Can you work these out from the model? Positions are in its coordinate system, mm. A direction names the side the tool comes from. Give positions to 0.01 mm unless a question says otherwise; leave off trailing zeros. Order: outer loops, then holes, each group sorted by start corner. A loop starts at its lowest first (then second) coordinate and runs counter-clockwise, first axis right, second up. Notation, with made-up numbers: (21.5, 8) -> (73.5, 8) arc R33 ccw to (73.5, 40) -> close; hole circle Ø4 at (-22.75, 46). An arc over 180 degrees is marked (long way). Answer as a JSON object with one key per item and string values.
```python
from build123d import *

# Parameters (mm, degrees)
F1_DEPTH = 3
F3_DEPTH = 7
F5_DEPTH = 4.7


with BuildPart() as f1:
    # F0 (on Top) → F1 (new body)
    with BuildSketch(Plane.XY):
        with BuildLine():
            Line((16.134871, -36.562502), (16.134871, -33.562502))
            Line((16.134871, -33.562502), (11.434871, -33.562502))
            Line((11.434871, -33.562502), (11.434871, -5.062502))
            ThreePointArc((11.434871, -5.062502), (10.849085, -3.648289), (9.434871, -3.062502))
            Line((9.434871, -3.062502), (5.084871, -3.062502))
            ThreePointArc((5.084871, -3.062502), (3.827619, -1.537502), (5.084871, -0.012502))
            Line((5.084871, -0.012502), (9.434871, -0.012502))
            ThreePointArc((9.434871, -0.012502), (10.849085, 0.573284), (11.434871, 1.987498))
            Line((11.434871, 1.987498), (11.434871, 30.487498))
            Line((11.434871, 30.487498), (16.134871, 30.487498))
            Line((16.134871, 30.487498), (16.134871, 33.487498))
            Line((16.134871, 33.487498), (8.634871, 33.487498))
            Line((8.634871, 33.487498), (5.20566, 5.305176))
            ThreePointArc((5.20566, 5.305176), (4.833466, 4.596348), (4.084871, 4.312498))
            Line((4.084871, 4.312498), (-9.615129, 4.312498))
            ThreePointArc((-9.615129, 4.312498), (-10.363724, 4.596348), (-10.735917, 5.305176))
            Line((-10.735917, 5.305176), (-14.165129, 33.487498))
            Line((-14.165129, 33.487498), (-21.665129, 33.487498))
            Line((-21.665129, 33.487498), (-21.665129, 30.487498))
            Line((-21.665129, 30.487498), (-16.965129, 30.487498))
            Line((-16.965129, 30.487498), (-16.965129, 1.987498))
            ThreePointArc((-16.965129, 1.987498), (-16.379342, 0.573284), (-14.965129, -0.012502))
            Line((-14.965129, -0.012502), (-10.615129, -0.012502))
            ThreePointArc((-10.615129, -0.012502), (-9.090129, -1.537502), (-10.615129, -3.062502))
            Line((-10.615129, -3.062502), (-14.965129, -3.062502))
            ThreePointArc((-14.965129, -3.062502), (-16.379342, -3.648289), (-16.965129, -5.062502))
            Line((-16.965129, -5.062502), (-16.965129, -33.562502))
            Line((-16.965129, -33.562502), (-21.665129, -33.562502))
            Line((-21.665129, -33.562502), (-21.665129, -36.562502))
            Line((-21.665129, -36.562502), (-14.165129, -36.562502))
            Line((-14.165129, -36.562502), (-10.742474, -9.904361))
            ThreePointArc((-10.742474, -9.904361), (-10.36591, -9.195764), (-9.615129, -8.912502))
            Line((-9.615129, -8.912502), (4.084871, -8.912502))
            ThreePointArc((4.084871, -8.912502), (4.835653, -9.195764), (5.212216, -9.904361))
            Line((5.212216, -9.904361), (8.634871, -36.562502))
            Line((8.634871, -36.562502), (16.134871, -36.562502))
        make_face()
    extrude(amount=F1_DEPTH)

    # F2 (on face) → F3 (join)
    with BuildSketch(Plane.XY.offset(3)):
        Polygon((-13.92177, 31.487498), (-16.965129, 31.487498), (-16.965129, 26.987498), (-13.374212, 26.987498), align=None)
        Polygon((11.434871, 26.987498), (11.434871, 31.487498), (8.391512, 31.487498), (7.843954, 26.987498), align=None)
    extrude(amount=F3_DEPTH)

    # F4 (on face) → F5 (cut)
    with BuildSketch(Plane.YZ.offset(16.134871)):
        with BuildLine():
            ThreePointArc((30.487498, 1.5), (30.926837, 2.56066), (31.987498, 3))
            Line((31.987498, 3), (30.487498, 3))
            Line((30.487498, 3), (30.487498, 1.5))
        make_face()
        with BuildLine():
            Line((30.487498, 0), (31.987498, 0))
            ThreePointArc((31.987498, 0), (30.926837, 0.43934), (30.487498, 1.5))
            Line((30.487498, 1.5), (30.487498, 0))
        make_face()
        with BuildLine():
            Line((33.487498, 0), (33.487498, 1.5))
            ThreePointArc((33.487498, 1.5), (33.048158, 0.43934), (31.987498, 0))
            Line((31.987498, 0), (33.487498, 0))
        make_face()
        with BuildLine():
            ThreePointArc((31.987498, 3), (33.048158, 2.56066), (33.487498, 1.5))
            Line((33.487498, 1.5), (33.487498, 3))
            Line((33.487498, 3), (31.987498, 3))
        make_face()
    extrude(amount=-F5_DEPTH, mode=Mode.SUBTRACT)


solid = f1.part
```
1. If we mould it in two halves opening along Y, with no side actions, what happens to faces 1 (the face through (-15, 29, 10)), 2 (the face through (10, 33.487, 1)), 3 (the face through (10, 26.987, 6)), 4 (the face through (-13, -0.013, 1))? For each: +Y half, -Y half, draft (parallel to the pull), parting line (faces both ways), or undercut.
Worked answers:
{"face 1": "draft", "face 2": "+Y half", "face 3": "-Y half", "face 4": "undercut"}
2. If we section it at C-C on x = -4.5: Please give me the cut outline in (y, z), then the cut area to 3 significant figures.
Worked answers:
{"outline": "(-8.91, 0) -> (4.31, 0) -> (4.31, 3) -> (-8.91, 3) -> close", "area": "39.7 mm²"}
3. Will these pins go through, and if not, where does the flat tip stop? pin 1 Ø12 at (x, y) = (-8, -2) entering from -Z; pin 2 Ø8 at (x, y) = (-13, 1.5) entering from +Z; pin 3 Ø1.1 at (x, z) = (-15.5, 7) entering from -Y; pin 4 Ø5 at (y, z) = (12, 3) entering from +X.
Worked answers:
{"pin 1": "z = 0", "pin 2": "z = 3", "pin 3": "y = 26.99", "pin 4": "x = 11.43"}
4. If we section it at A-A on y = -32: Please give me the cut outline in (x, z).
Worked answers:
{"outline": "(-16.97, 0) -> (-13.58, 0) -> (-13.58, 3) -> (-16.97, 3) -> close; (8.05, 0) -> (11.43, 0) -> (11.43, 3) -> (8.05, 3) -> close"}
5. If we section it at B-B on z = 5.75: Please give me the cut outline in (x, y), then the cut area to 3 significant figures.
Worked answers:
{"outline": "(-16.97, 26.99) -> (-13.37, 26.99) -> (-13.92, 31.49) -> (-16.97, 31.49) -> close; (7.84, 26.99) -> (11.43, 26.99) -> (11.43, 31.49) -> (8.39, 31.49) -> close", "area": "29.9 mm²"}
6. For faces 5 (the face through (10.9, -3.7, 1.5)), 6 (the face through (11.435, 33.12, 2.7)), 7 (the face through (-16.36, -3.63, 1.48)), 8 (the face through (-15, 31.487, 6)), which set-ups out of +Z, -Z, +X, -X, +Y, -Y let a thin tool reach every point of the face, with its end or its side?
Worked answers:
{"face 5": "+Z, -Z, +X", "face 6": "+Z, +X, +Y", "face 7": "+Z, -Z, -X", "face 8": "+Z, +X, -X, +Y"}
7. Please list where these lines run through material, in increasing order: L1, parallel to Y at x = 9, z = 2.75; L2, parallel to X at y = -30.5, z = 2.25; L3, parallel to Y at x = -15, z = 3.75.
Worked answers:
{"L1": "-36.56 to -3.06, -0.01 to 33.49", "L2": "-16.97 to -13.39, 7.86 to 11.43", "L3": "26.99 to 31.49"}
